Check sheet for the drawn part. Datum: minimum x, y, z corner. Units: mm. Coordinates: 2 decimals unless noted, no trailing zeros. Write each loop counter-clockwise with the first axis right and the second up, starting at its lowest first coordinate (ties: lowest second). Pieces come first, ordered by that corner, then holes. Notation, with made-up numbers: (-35.5, 53.25) -> (-20.5, 53.25) arc R31 cw to (-20.5, 84.25) -> close; hole circle Ø10 at (33, 62). An arc over 180 degrees is marked (long way). Answer in a Markdown table with one row per item.
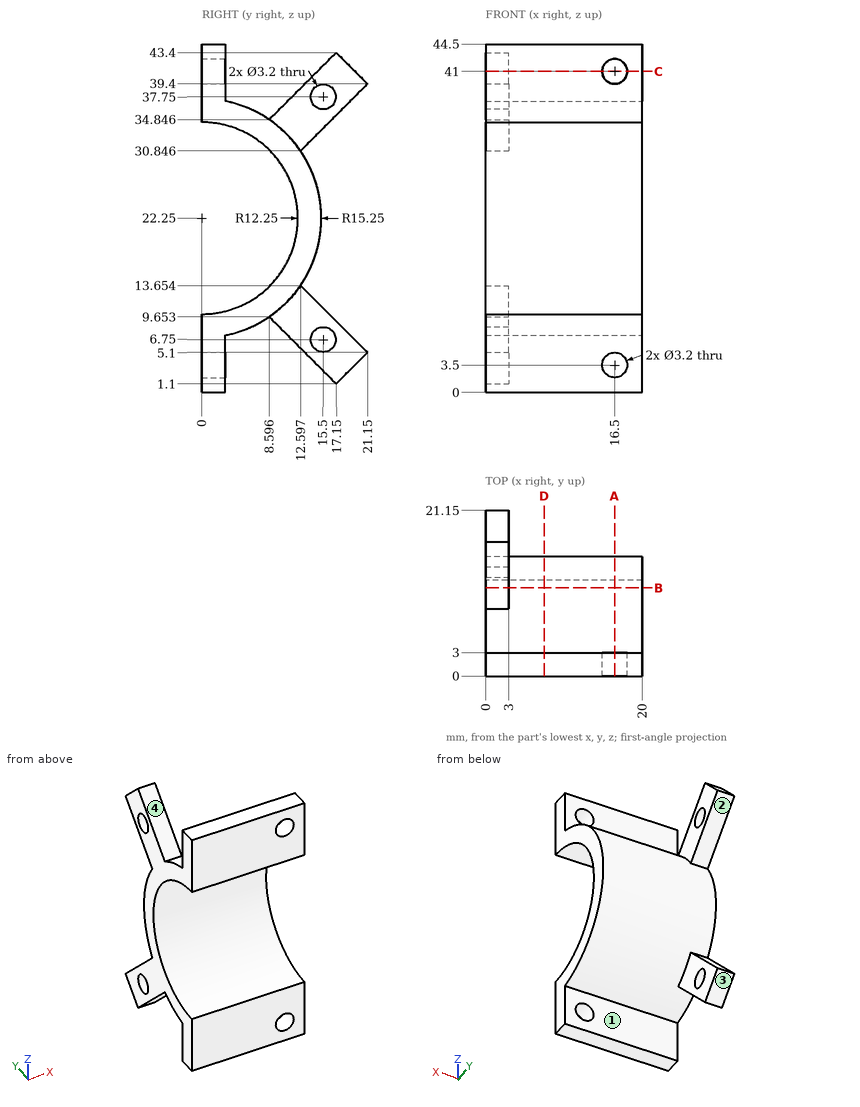
1. Sectioned sample at C-C, the plane z = 41. Record the cut outline in (x, y).
Findings below:
| item | result |
|---|---|
| outline | (0, 0) -> (14.9, 0) -> (14.9, 3) -> (0, 3) -> close; (0, 14.75) -> (3, 14.75) -> (3, 19.55) -> (0, 19.55) -> close; (18.1, 0) -> (20, 0) -> (20, 3) -> (18.1, 3) -> close |
2. Sectioned sample at B-B, the plane y = 11.25. Record the cut outline in (x, z) (1 decimal).
Findings below:
| item | result |
|---|---|
| outline | (0, 7) -> (3, 7) -> (3, 12) -> (20, 12) -> (20, 17.4) -> (0, 17.4) -> close; (0, 27.1) -> (20, 27.1) -> (20, 32.5) -> (3, 32.5) -> (3, 37.5) -> (0, 37.5) -> close |
3. Sectioned sample at D-D, the plane x = 7.5. Record the cut outline in (y, z).
Findings below:
| item | result |
|---|---|
| outline | (0, 0) -> (3, 0) -> (3, 7.3) arc R15.25 ccw to (3, 37.2) -> (3, 44.5) -> (0, 44.5) -> (0, 34.5) arc R12.25 cw to (0, 10) -> close |
4. Go/stop test with flat-tipped pins: pin 1 (2 mm diameter, centred on x = 11, y = 11.5, fed in from +Z); pin 2 (2 mm diameter, centred on x = 8.5, z = 34, fed in from +Y) (1 decimal); pin 3 (4 mm diameter, centred on y = 15.5, z = 37.75, fed in from +X); pin 4 (3 mm diameter, centred on y = 15.5, z = 6.75, fed in from -X). Record where each tip stops, or that it passes through.
Findings below:
| item | result |
|---|---|
| pin 1 | stops at z = 33.31 |
| pin 2 | stops at y = 10.8 |
| pin 3 | stops at x = 3 |
| pin 4 | passes through |
5. Release check for a two-part mould opening along Z. For the marked faces 1, 2, 3 and 4 record: released by +Z, released by -Z, zero draft, split by the parting line, or undercut.
Findings below:
| item | result |
|---|---|
| face 1 | zero draft |
| face 2 | undercut |
| face 3 | released by -Z |
| face 4 | released by +Z |
6. Sectioned sample at A-A, the plane x = 16.5. Record the cut outline in (y, z), and give its area (3 significant figures).
Findings below:
| item | result |
|---|---|
| outline | (0, 0) -> (3, 0) -> (3, 1.9) -> (0, 1.9) -> close; (0, 5.1) -> (3, 5.1) -> (3, 7.3) arc R15.25 ccw to (3, 37.2) -> (3, 39.4) -> (0, 39.4) -> (0, 34.5) arc R12.25 cw to (0, 10) -> close; (0, 42.6) -> (3, 42.6) -> (3, 44.5) -> (0, 44.5) -> close |
| area | 153 mm² |
7. Material ranges on probe 1 along X at (y, z) = (0.9, 41); probe 2 along Z at (x, y) = (16.5, 1); probe 3 along Z at (x, y) = (16.5, 1.75) (1 decimal), recorded low to high. Write a range as from..to.
Findings below:
| item | result |
|---|---|
| probe 1 | x = 0..14.9, 18.1..20 |
| probe 2 | z = 0..1.9, 5.1..10.04, 34.46..39.4, 42.6..44.5 |
| probe 3 | z = 0..1.9, 5.1..10.1, 34.4..39.4, 42.6..44.5 |
